Could you check a few things on this model? Use its own coordinates, in mm. Coordinates: 2 decimals unless noted, no trailing zeros. Order: outer loops, then holes, each group sorted by start corner. A loop starts at its lowest first (then second) coordinate and runs counter-clockwise, first axis right, second up. Notation, with made-up numbers: (52.5, 14) - (62.5, 14) arc R21 cw to (62.5, 47) - close; hole circle Ø7 at (-35.75, -6.75). An arc over 180 degrees is marked (long way). One line per item, written item: value.
from build123d import *

# Parameters (mm, degrees)
PAD015_DEPTH                        = 3
SKETCH054_R                         = 1.65
POCKET018_DEPTH                     = 358.938883
POCKET018_DEPTH_BACK                = 361.938883
BODY001003005003004_PLACEMENT_ANGLE = 60
CLONE027_PLACEMENT_ANGLE            = 60


with BuildPart() as part:
    # Sketch053 → Pad015 (new body)
    with BuildSketch(Plane.XY):
        with BuildLine():
            ThreePointArc((152.005097, 113.785532), (84.992984, 169.790723), (0, 189.875477))
            Line((0, 189.875477), (0, 196.875477))
            ThreePointArc((157.608957, 117.98038), (88.126358, 176.050273), (0, 196.875477))
            ThreePointArc((152.005097, 113.785532), (156.904451, 113.081026), (157.608957, 117.98038))
        make_face()
    pad015 = extrude(amount=PAD015_DEPTH)

    # Sketch054 → Pocket018 (cut, two sides)
    with BuildSketch(Plane.XY) as pocket018_sk:
        with Locations((150.82443, 121.020933)):
            Circle(SKETCH054_R)
        with BuildLine():
            ThreePointArc((0, 191.725477), (1.65, 193.375477), (0, 195.025477))
            Line((0, 191.725477), (0, 195.025477))
        make_face()
    pocket018 = extrude(amount=-POCKET018_DEPTH, mode=Mode.SUBTRACT) + extrude(pocket018_sk.sketch, amount=POCKET018_DEPTH_BACK, mode=Mode.SUBTRACT)

    # Mirrored020: Pad015, Pocket018 across Sketch053 V_Axis
    add(pad015.mirror(Plane(origin=(0, 0, 0), x_dir=(0, 0, 1), z_dir=(1, 0, 0))))
    add(pocket018.mirror(Plane(origin=(0, 0, 0), x_dir=(0, 0, 1), z_dir=(1, 0, 0))), mode=Mode.SUBTRACT)


with BuildPart() as part_1:
    # Body001003005003004 placement: moved
    add(part.part.rotate(Axis((0, 0, 0), (0, 0, 1)), BODY001003005003004_PLACEMENT_ANGLE))


with BuildPart() as part_2:
    # Clone027 placement: moved
    add(part_1.part.moved(Location((0, -83, 0))).rotate(Axis((0, -83, 0), (0, 0, -1)), CLONE027_PLACEMENT_ANGLE))


solid = part_2.part
Item 1: I'm going to push flat-ended pins straight in: pin 1 Ø3 at (x, y) = (150.82, 38.02) entering from +Z; pin 2 Ø1.5 at (x, z) = (-101.5, 2.5) entering from +Y. Where does each tip first touch, or does it pass through?
Conclusion:
pin 1: through
pin 2: y = 86.14
Item 2: I want a section at B-B on z = 1.75. Please give me the cut outline in (x, y).
Conclusion:
outline: (-157.61, 34.98) arc R3.5 ccw to (-152.01, 30.79) arc R189.88 cw to (0, 106.88) arc R189.88 cw to (152.01, 30.79) arc R3.5 ccw to (157.61, 34.98) arc R196.88 ccw to (0, 113.88) arc R196.88 ccw to start; hole circle Ø3.3 at (-150.82, 38.02); hole circle Ø3.3 at (0, 110.38); hole circle Ø3.3 at (150.82, 38.02)
Item 3: I want a section at A-A on y = 96.5. Please give me the cut outline in (x, z), then the cut area to 3 significant figures.
Conclusion:
outline: (-80.87, 0) - (-61.91, 0) - (-61.91, 3) - (-80.87, 3) - close; (61.91, 0) - (80.87, 0) - (80.87, 3) - (61.91, 3) - close
area: 114 mm²
Item 4: If I drill on probe 1 along X at (y, z) = (53.5, 2.5); probe 2 along X at (y, z) = (76, 2.15); probe 3 along Y at (x, z) = (49.5, 2.7), over which ranges is the centre line in solid material (lowest first)?
Conclusion:
probe 1: -141.87 to -131.99, 131.99 to 141.87
probe 2: -116.1 to -103.79, 103.79 to 116.1
probe 3: 100.31 to 107.55
Item 5: I want a section at C-C on y = 59. Please give me the cut outline in (x, z), then the cut area to 3 significant figures.
Conclusion:
outline: (-136.37, 0) - (-126.05, 0) - (-126.05, 3) - (-136.37, 3) - close; (126.05, 0) - (136.37, 0) - (136.37, 3) - (126.05, 3) - close
area: 61.9 mm²
Item 6: Thinking about a two-plate mould opening in X: for faces 1 (the face through (156.842, 30.036, 1.479)), 2 (the face through (-12, 109, 0)), 3 (the face through (-156.842, 30.036, 1.479)), which applies, pulls with the +X half, pulls with the -X half, needs draft (parallel to the pull), parting line crosses it, or undercut?
Conclusion:
face 1: undercut
face 2: needs draft
face 3: undercut
Item 7: I want a section at D-D on x = -18. Please give me the cut outline in (y, z).
Conclusion:
outline: (106.02, 0) - (113.05, 0) - (113.05, 3) - (106.02, 3) - close
